```python
from build123d import *

# Parameters (mm, degrees)
SKETCH_1_R               = 8
EXTRUDE_1_DEPTH          = 16
SKETCH_2_R               = 4
CUT_EXTRUDE_1_DEPTH      = 20.595917942
SKETCH_3_OUTSIDE_W       = 23.542
SKETCH_3_OUTSIDE_H       = 23.542
SKETCH_3_OUTSIDE_R       = 6.5
CUT_EXTRUDE_2_DEPTH      = 6
CUT_EXTRUDE_3_DEPTH      = 20.595917942
CUT_EXTRUDE_3_DEPTH_BACK = 20.595917942
SKETCH_4_R               = 1.5
CUT_EXTRUDE_4_DEPTH      = 20.595918116
CUT_EXTRUDE_4_DEPTH_BACK = 20.595918116
SKETCH_5_R               = 1.5


with BuildPart() as part:
    # 草图1 → 凸台-拉伸1 (new body)
    with BuildSketch(Plane(origin=(0, 0, 0), x_dir=(1, 0, 0), z_dir=(0, 1, 0))):
        with Locations(Location((0, 0, 0), (0, 0, 270))):
            Circle(SKETCH_1_R)
    extrude(amount=EXTRUDE_1_DEPTH)

    # 草图2 → 切除-拉伸1 (cut, through all)
    with BuildSketch(Plane(origin=(0, 16, 0), x_dir=(1, 0, 0), z_dir=(0, 1, 0))):
        with Locations(Location((0, 0, 0), (0, 0, 270))):
            Circle(SKETCH_2_R)
    extrude(amount=-CUT_EXTRUDE_1_DEPTH, mode=Mode.SUBTRACT)

    # 草图3 outside → 切除-拉伸2 (cut)
    with BuildSketch(Plane(origin=(0, 3, 0), x_dir=(1, 0, 0), z_dir=(0, 1, 0))):
        Rectangle(SKETCH_3_OUTSIDE_W, SKETCH_3_OUTSIDE_H)
        with Locations(Location((0, 0, 0), (0, 0, 270))):
            Circle(SKETCH_3_OUTSIDE_R, mode=Mode.SUBTRACT)
    extrude(amount=CUT_EXTRUDE_2_DEPTH, mode=Mode.SUBTRACT)

    # 草图4 → 切除-拉伸3 (cut, two sides: drawn at the far end of the back side and taken through both)
    with BuildSketch(Plane(origin=(0, 0, 0), x_dir=(0, 0, -1), z_dir=(1, 0, 0)).offset(-CUT_EXTRUDE_3_DEPTH_BACK)):
        with Locations((0, 12.5)):
            Circle(SKETCH_4_R)
    extrude(amount=CUT_EXTRUDE_3_DEPTH + CUT_EXTRUDE_3_DEPTH_BACK, mode=Mode.SUBTRACT)

    # 草图5 → 切除-拉伸4 (cut, two sides: drawn at the far end of the back side and taken through both)
    with BuildSketch(Plane.XY.offset(-CUT_EXTRUDE_4_DEPTH_BACK)):
        with Locations((0, 12.5)):
            Circle(SKETCH_5_R)
    extrude(amount=CUT_EXTRUDE_4_DEPTH + CUT_EXTRUDE_4_DEPTH_BACK, mode=Mode.SUBTRACT)


solid = part.part
```
Model file for the job. Use its own axes, mm. A direction names the side the tool comes from. Give positions to 0.01 mm unless a question says otherwise; leave off trailing zeros. Write each loop counter-clockwise with the first axis right and the second up, starting at its lowest first coordinate (ties: lowest second). Pieces come first, ordered by that corner, then holes. Notation, with made-up numbers: (32.5, 81) - (64.5, 81) arc R14 cw to (64.5, 94) - close; hole circle Ø2 at (-33, -34.75). An arc over 180 degrees is marked (long way). One line per question, with ' | ' between items. Start each with the question number.
(1) Slice it at C-C on y = 2.5. Write the cut outline in (x, z), plus the area to 3 significant figures.
(2) Slice it at D-D on z = -6.25. Write the cut outline in (x, y), plus the area to 3 significant figures.
(3) Pin check, flat tips, straight feed: P1, Ø6, axis at y = 12.5, z = -4.5, coming from the -X side; P2, Ø1, axis at x = 0.5, y = 5.5, coming from the +Z side; P3, Ø6, axis at x = -4.5, y = 13, coming from the +Z side. Stop position of each tip, or through.
(4) Slice it at A-A on x = 0. Write the cut outline in (y, z).
(5) Two-plate mould, pull along Y, no slides. Class faces 1 (the face through (-2, 16, -4)), 2 (the face through (1.386, 11.925, -5.885)), 3 (the face through (-7.81, 1.48, -1.73)): +Y half, -Y half, draft (parallel to the pull), parting line (faces both ways), or undercut.
(6) 3-axis set-ups, long thin cutter, end or side, ignore diameter. For faces 4 (the face through (-1.532, 8.112, 3.695)), 5 (the face through (0, 9, -7)): which of +Z, -Z, +X, -X, +Y, -Y reach the whole face in a straight line?
(7) Slice it at B-B on z = 0. Write the cut outline in (x, y), plus the area to 3 significant figures.
(8) Wall check: line 1 along Y through (x, z) = (0, 6.9); line 2 along X through (y, z) = (5.5, 0); line 3 along Y through (x, z) = (7, -3). Give the ranges that are in metal, low to high. Write a range as from..to.
Results below:
1) outline: circle Ø16 at (0, 0); hole circle Ø8 at (0, 0) | area: 151 mm^2
2) outline: (-4.99, 0) - (4.99, 0) - (4.99, 3) - (1.79, 3) - (1.79, 9) - (4.99, 9) - (4.99, 16) - (-4.99, 16) - (-4.99, 9) - (-1.79, 9) - (-1.79, 3) - (-4.99, 3) - close; hole circle Ø3 at (0, 12.5) | area: 114 mm^2
3) P1: x = -7.86 | P2: z = 6.5 | P3: z = 7.86
4) outline: (0, -8) - (3, -8) - (3, -6.5) - (9, -6.5) - (9, -8) - (11, -8) - (11, -4) - (0, -4) - close; (0, 4) - (11, 4) - (11, 8) - (9, 8) - (9, 6.5) - (3, 6.5) - (3, 8) - (0, 8) - close; (14, -8) - (16, -8) - (16, -4) - (14, -4) - close; (14, 4) - (16, 4) - (16, 8) - (14, 8) - close
5) face 1: +Y half | face 2: undercut | face 3: draft
6) face 4: +Y, -Y | face 5: none
7) outline: (-8, 0) - (-4, 0) - (-4, 11) - (-8, 11) - (-8, 9) - (-6.5, 9) - (-6.5, 3) - (-8, 3) - close; (-8, 14) - (-4, 14) - (-4, 16) - (-8, 16) - close; (4, 0) - (8, 0) - (8, 3) - (6.5, 3) - (6.5, 9) - (8, 9) - (8, 11) - (4, 11) - close; (4, 14) - (8, 14) - (8, 16) - (4, 16) - close | area: 86.0 mm^2
8) line 1: 0..3, 9..11, 14..16 | line 2: -6.5..-4, 4..6.5 | line 3: 0..3, 9..16
